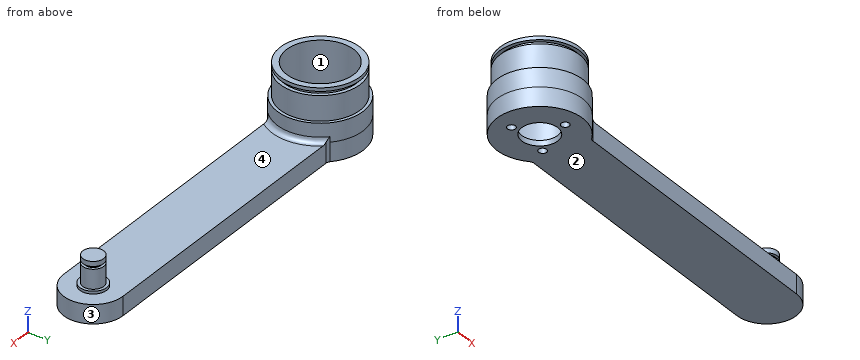
from build123d import *

# Parameters (mm, degrees)
EXTRUDE_1_DEPTH     = 7
SKETCH_2_R          = 6.7
CUT_EXTRUDE_1_DEPTH = 7
SKETCH_3_R          = 12.5
SKETCH_3_R_2        = 6.7
CUT_EXTRUDE_2_DEPTH = 5
SKETCH_4_R          = 16
SKETCH_4_R_2        = 12.5
EXTRUDE_2_DEPTH     = 7
SKETCH_5_R          = 14.85
SKETCH_5_R_2        = 12.5
EXTRUDE_3_DEPTH     = 12
SKETCH_6_R          = 5
EXTRUDE_4_DEPTH     = 1
SKETCH_7_R          = 3.9
EXTRUDE_5_DEPTH     = 10
FILLET_1_R          = 2
SKETCH_8_R          = 1.5
CUT_EXTRUDE_3_DEPTH = 10
SKETCH_9_R          = 14.85
SKETCH_9_R_2        = 13.5
CUT_EXTRUDE_4_DEPTH = 1.5
SKETCH_10_R         = 3.9
SKETCH_10_R_2       = 2.9
CUT_EXTRUDE_5_DEPTH = 1


with BuildPart() as part:
    # Sketch 1 → Extrude 1 (new body)
    with BuildSketch(Plane.XY):
        with BuildLine():
            Line((119.609580579, 11), (11.618950039, 11))
            ThreePointArc((11.618950039, 11), (-16, 0), (11.618950039, -11))
            Line((11.618950039, -11), (119.609580579, -11))
            ThreePointArc((119.609580579, -11), (130.609580579, 0), (119.609580579, 11))
        make_face()
    extrude(amount=EXTRUDE_1_DEPTH)

    # Sketch 2 → Cut-Extrude 1 (cut)
    with BuildSketch(Plane.XY.offset(7)):
        Circle(SKETCH_2_R)
    extrude(amount=-CUT_EXTRUDE_1_DEPTH, mode=Mode.SUBTRACT)

    # Sketch 3 → Cut-Extrude 2 (cut)
    with BuildSketch(Plane.XY.offset(7)):
        Circle(SKETCH_3_R)
        Circle(SKETCH_3_R_2, mode=Mode.SUBTRACT)
    extrude(amount=-CUT_EXTRUDE_2_DEPTH, mode=Mode.SUBTRACT)

    # Sketch 4 → Extrude 2 (add)
    with BuildSketch(Plane.XY.offset(7)):
        with Locations(Location((0, 0, 0), (0, 0, 316.567463442))):
            Circle(SKETCH_4_R)
        Circle(SKETCH_4_R_2, mode=Mode.SUBTRACT)
    extrude(amount=EXTRUDE_2_DEPTH)

    # Sketch 5 → Extrude 3 (add)
    with BuildSketch(Plane.XY.offset(14)):
        Circle(SKETCH_5_R)
        Circle(SKETCH_5_R_2, mode=Mode.SUBTRACT)
    extrude(amount=EXTRUDE_3_DEPTH)

    # Sketch 6 → Extrude 4 (add)
    with BuildSketch(Plane.XY.offset(7)):
        with Locations((119.609580579, 0)):
            Circle(SKETCH_6_R)
    extrude(amount=EXTRUDE_4_DEPTH)

    # Sketch 7 → Extrude 5 (add)
    with BuildSketch(Plane.XY.offset(8)):
        with Locations((119.609580579, 0)):
            Circle(SKETCH_7_R)
    extrude(amount=EXTRUDE_5_DEPTH)

    # Fillet 1
    # the kernel refuses this fillet: 2 mm, written as the material it adds along each edge
    with BuildSketch(Plane(origin=(0, 0, 7), x_dir=(0.47954718697037524, -0.8775160941366261, 0), z_dir=(-0.8775160941366261, -0.47954718697037524, 0))) as fillet_1_piece_1_section:
        with BuildLine():
            CenterArc((16 + FILLET_1_R, FILLET_1_R), FILLET_1_R, 180, 90)
            Line((16 + FILLET_1_R, 0), (16, 0))
            Line((16, 0), (16, FILLET_1_R))
        make_face()
    fillet_1_piece_1 = revolve(axis=Axis((0, 0, 7), (0, 0, 1)), revolution_arc=122.688335481, mode=Mode.PRIVATE)
    fillet_1_piece_1 = split(fillet_1_piece_1, bisect_by=Plane(origin=(16.565225079, -11, 7.565225079), z_dir=(0, 1, 0)), keep=Keep.TOP, mode=Mode.PRIVATE)
    fillet_1_piece_1 = split(fillet_1_piece_1, bisect_by=Plane(origin=(16.565225079, 11, 7.565225079), z_dir=(0, -1, 0)), keep=Keep.TOP, mode=Mode.PRIVATE)
    add(fillet_1_piece_1)
    with BuildSketch(Plane(origin=(11.618950039, -11, 0), x_dir=(1, 0, 0), z_dir=(0, 0, 1))) as fillet_1_piece_2:
        with BuildLine():
            CenterArc((0.830949559, -2), FILLET_1_R, 90, 43.761742693)
            ThreePointArc((-0.552372618, -0.555555556), (-0.27278551, -0.281159093), (0, 0))
            Line((0, 0), (0.830949559, 0))
        make_face()
    extrude(amount=7)
    with BuildSketch(Plane(origin=(11.618950039, 11, 0), x_dir=(-0.7050724433144171, 0.7091352830586264, 0), z_dir=(0, 0, 1))) as fillet_1_piece_3:
        with BuildLine():
            CenterArc((0.83239093, -1.999400538), FILLET_1_R, 91.402860375, 43.761742693)
            Line((-0.585879636, -0.589255651), (0, 0))
            ThreePointArc((0, 0), (0.391713379, -0.004795699), (0.783426758, 0))
        make_face()
    extrude(amount=7)
    with BuildSketch(Plane(origin=(11.618950039, -11, 0), x_dir=(1, 0, 0), z_dir=(0, 0, 1))) as fillet_1_piece_4a_section:
        with BuildLine():
            CenterArc((0.830949559, -2), FILLET_1_R, 90, 43.761742693)
            ThreePointArc((-0.552372618, -0.555555556), (-0.27278551, -0.281159093), (0, 0))
            Line((0, 0), (0.830949559, 0))
        make_face()
    fillet_1_piece_4a = extrude(amount=9.077373898, mode=Mode.PRIVATE)
    fillet_1_piece_4a = split(fillet_1_piece_4a, bisect_by=Plane(origin=(11.685470733, -11.116370602, 7), z_dir=(0, 0, 1)), keep=Keep.TOP, mode=Mode.PRIVATE)
    with BuildSketch(Plane(origin=(0, 0, 7), x_dir=(0.47954718697037524, -0.8775160941366261, 0), z_dir=(-0.8775160941366261, -0.47954718697037524, 0))) as fillet_1_piece_4b_section:
        with BuildLine():
            CenterArc((16 + FILLET_1_R, FILLET_1_R), FILLET_1_R, 180, 90)
            Line((16 + FILLET_1_R, 0), (16, 0))
            Line((16, 0), (16, FILLET_1_R))
        make_face()
    fillet_1_piece_4b = revolve(axis=Axis((0, 0, 7), (0, 0, 1)), revolution_arc=122.688335481, mode=Mode.PRIVATE)
    fillet_1_piece_4b = split(fillet_1_piece_4b, bisect_by=Plane(origin=(10.195969893, -11, 7.42845241), z_dir=(0, -1, 0)), keep=Keep.TOP, mode=Mode.PRIVATE)
    fillet_1_piece_4 = fillet_1_piece_4a & fillet_1_piece_4b
    add(fillet_1_piece_4)
    with BuildSketch(Plane(origin=(11.618950039, 11, 0), x_dir=(-0.7050724433144171, 0.7091352830586264, 0), z_dir=(0, 0, 1))) as fillet_1_piece_5a_section:
        with BuildLine():
            CenterArc((0.83239093, -1.999400538), FILLET_1_R, 91.402860375, 43.761742693)
            Line((-0.585879636, -0.589255651), (0, 0))
            ThreePointArc((0, 0), (0.391713379, -0.004795699), (0.783426758, 0))
        make_face()
    fillet_1_piece_5a = extrude(amount=9.077373898, mode=Mode.PRIVATE)
    fillet_1_piece_5a = split(fillet_1_piece_5a, bisect_by=Plane(origin=(11.685470733, 11.116370602, 7), z_dir=(0, 0, 1)), keep=Keep.TOP, mode=Mode.PRIVATE)
    with BuildSketch(Plane(origin=(0, 0, 7), x_dir=(0.47954718697037524, -0.8775160941366261, 0), z_dir=(-0.8775160941366261, -0.47954718697037524, 0))) as fillet_1_piece_5b_section:
        with BuildLine():
            CenterArc((16 + FILLET_1_R, FILLET_1_R), FILLET_1_R, 180, 90)
            Line((16 + FILLET_1_R, 0), (16, 0))
            Line((16, 0), (16, FILLET_1_R))
        make_face()
    fillet_1_piece_5b = revolve(axis=Axis((0, 0, 7), (0, 0, 1)), revolution_arc=122.688335481, mode=Mode.PRIVATE)
    fillet_1_piece_5b = split(fillet_1_piece_5b, bisect_by=Plane(origin=(10.195969605, 11, 7.428452615), z_dir=(0, 1, 0)), keep=Keep.TOP, mode=Mode.PRIVATE)
    fillet_1_piece_5 = fillet_1_piece_5a & fillet_1_piece_5b
    add(fillet_1_piece_5)

    # Sketch 8 → Cut-Extrude 3 (cut)
    with BuildSketch(Plane(origin=(0, 0, 0), x_dir=(-1, 0, 0), z_dir=(0, 0, -1))):
        with Locations((0, -9.5)):
            Circle(SKETCH_8_R)
        with Locations((-8.227241336, 4.75)):
            Circle(SKETCH_8_R)
        with Locations((8.227241336, 4.75)):
            Circle(SKETCH_8_R)
    extrude(amount=-CUT_EXTRUDE_3_DEPTH, mode=Mode.SUBTRACT)

    # Sketch 9 → Cut-Extrude 4 (cut)
    with BuildSketch(Plane.XY.offset(23.2)):
        Circle(SKETCH_9_R)
        Circle(SKETCH_9_R_2, mode=Mode.SUBTRACT)
    extrude(amount=CUT_EXTRUDE_4_DEPTH, mode=Mode.SUBTRACT)

    # Sketch 10 → Cut-Extrude 5 (cut)
    with BuildSketch(Plane.XY.offset(15.2)):
        with Locations((119.609580579, 0)):
            Circle(SKETCH_10_R)
        with Locations((119.609580579, 0)):
            Circle(SKETCH_10_R_2, mode=Mode.SUBTRACT)
    extrude(amount=CUT_EXTRUDE_5_DEPTH, mode=Mode.SUBTRACT)


solid = part.part
Source: CAD feature listing. Evaluate the final solid. Frame: model axes, mm. Face numbers are marked on the shaded views. Round coordinates to 2 decimals unless told otherwise and drop trailing zeros. Loops run counter-clockwise (first coordinate to the right, second up) from the corner with the lowest first, then second, coordinate; pieces in that order, holes last. Notation, with made-up numbers: (4, 53) - (15, 53) arc R26 cw to (15, 83) - close; hole circle Ø7 at (84, 66). An arc over 180 degrees is marked (long way). Write item = value, one per line. Start each with the question number.
(1) Section query A-A, the plane x = 0. Output: boundary loops of the cut face in (y, z), plus the area to 3 significant figures.
(2) Ray query, line 1 along Z through (x, y) = (122, -3); line 2 along Z through (x, y) = (62, 7); line 3 along Y through (x, z) = (55.5, 2.25). Return the intervals inside material, ascending. Write a range as from..to.
(3) Section query B-B, the plane z = 11. Output: boundary loops of the cut face in (x, y).
(4) Pin query (flat end, axial travel): pin 1 (3 mm diameter, centred on x = 58, z = 4.5, fed in from +Y); pin 2 (4 mm diameter, centred on x = 99.5, y = -3.5, fed in from +Z); pin 3 (2.5 mm diameter, centred on x = 79, z = 4, fed in from -Y). Return the tip coordinate at first contact, or that it passes through.
(5) Section query C-C, the plane x = 44. Output: boundary loops of the cut face in (y, z).
(6) Pull-direction query (X, two-part tool) for the marked faces 1, 2, 3 and 4; classes: +X half, -X half, draft (parallel to the pull), parting line (faces both ways), or undercut.
Conclusion:
q1.outline = (-16, 0) - (-11, 0) - (-11, 2) - (-12.5, 2) - (-12.5, 26) - (-14.85, 26) - (-14.85, 24.7) - (-13.5, 24.7) - (-13.5, 23.2) - (-14.85, 23.2) - (-14.85, 14) - (-16, 14) - close; (-8, 0) - (-6.7, 0) - (-6.7, 2) - (-8, 2) - close; (6.7, 0) - (16, 0) - (16, 14) - (14.85, 14) - (14.85, 23.2) - (13.5, 23.2) - (13.5, 24.7) - (14.85, 24.7) - (14.85, 26) - (12.5, 26) - (12.5, 2) - (6.7, 2) - close
q1.area = 168 mm2
q2.line_1 = 0..15.2, 16.2..18
q2.line_2 = 0..7
q2.line_3 = -11..11
q3.outline = circle Ø32 at (0, 0); circle Ø7.8 at (119.61, 0); hole circle Ø25 at (0, 0)
q4.pin_1 = 11
q4.pin_2 = 7
q4.pin_3 = -11
q5.outline = (-11, 0) - (11, 0) - (11, 7) - (-11, 7) - close
q6.face_1 = undercut
q6.face_2 = draft
q6.face_3 = +X half
q6.face_4 = undercut
